```python
from build123d import *

# Parameters (mm, degrees)
SKETCH1_W_MOCK_PCB_W     = 63.5
SKETCH1_W_MOCK_PCB_H     = 209.042
BOSS_EXTRUDE1_DEPTH      = 6.35
F_5_16_CLEARANCE_HOLE1_D = 8.4328
CUT_EXTRUDE1_DEPTH       = 13.7


with BuildPart() as part:
    # Sketch1 w/mock PCB → Boss-Extrude1 (new body, symmetric)
    with BuildSketch(Plane.XY):
        Rectangle(SKETCH1_W_MOCK_PCB_W, SKETCH1_W_MOCK_PCB_H)
    extrude(amount=BOSS_EXTRUDE1_DEPTH, both=True)

    # 5/16 Clearance Hole1 (through all)
    with Locations(Plane.XY.offset(6.35)):
        with Locations((-19.05, -94.869), (19.05, -94.869)):
            Hole(F_5_16_CLEARANCE_HOLE1_D / 2)

    # Sketch3 → Cut-Extrude1 (cut, through all)
    with BuildSketch(Plane.XY.offset(6.35)):
        with BuildLine():
            Line((-23.2664, 93.599), (-23.2664, 96.139))
            ThreePointArc((-23.2664, 96.139), (-19.05, 100.3554), (-14.8336, 96.139))
            Line((-14.8336, 96.139), (-14.8336, 93.599))
            ThreePointArc((-14.8336, 93.599), (-19.05, 89.3826), (-23.2664, 93.599))
        make_face()
        with BuildLine():
            Line((23.2664, 93.599), (23.2664, 96.139))
            ThreePointArc((23.2664, 96.139), (19.05, 100.3554), (14.8336, 96.139))
            Line((14.8336, 96.139), (14.8336, 93.599))
            ThreePointArc((14.8336, 93.599), (19.05, 89.3826), (23.2664, 93.599))
        make_face()
    extrude(amount=-CUT_EXTRUDE1_DEPTH, mode=Mode.SUBTRACT)


solid = part.part
```
CAD build for the part. Positions are in the model's coordinates, mm. A direction names the side the tool comes from. Coordinates: 2 decimals unless noted, no trailing zeros. Order: outer loops, then holes, each group sorted by start corner. A loop starts at its lowest first (then second) coordinate and runs counter-clockwise, first axis right, second up.
(1) Saw through at B-B, the plane x = 20.5. Write the cut outline in (y, z).
Solution:
outline: (-104.52, -6.35) - (-98.83, -6.35) - (-98.83, 6.35) - (-104.52, 6.35) - close; (-90.91, -6.35) - (89.64, -6.35) - (89.64, 6.35) - (-90.91, 6.35) - close; (100.1, -6.35) - (104.52, -6.35) - (104.52, 6.35) - (100.1, 6.35) - close
(2) Which spindle directions (+Z, -Z, +X, -X, +Y, -Y) get a long thin tool onto all of the face, cutting with end or side? Do faces 1 (the face through (-18.957, 89.384, 0.089)), 2 (the face through (-31.75, -1, 0)). Say none if no direction does.
Solution:
face 1: +Z, -Z
face 2: +Z, -Z, -X, +Y, -Y
(3) Drill centre lines: L1, parallel to Y at x = -19.05, z = 3.25; L2, parallel to Y at x = -19.5, z = -5.5. Where is each one in solid material? Low to high.
Solution:
L1: y = -104.52 to -99.09, -90.65 to 89.38, 100.36 to 104.52
L2: y = -104.52 to -99.06, -90.68 to 89.41, 100.33 to 104.52
(4) Pin check, flat tip, straight feed: pin 1 Ø6.5 at (x, y) = (-19.05, -94.869) entering from -Z. Stop position of the tip, or through.
Solution:
pin 1: passes through
(5) Saw through at A-A, the plane x = -19.05. Write the cut outline in (y, z).
Solution:
outline: (-104.52, -6.35) - (-99.09, -6.35) - (-99.09, 6.35) - (-104.52, 6.35) - close; (-90.65, -6.35) - (89.38, -6.35) - (89.38, 6.35) - (-90.65, 6.35) - close; (100.36, -6.35) - (104.52, -6.35) - (104.52, 6.35) - (100.36, 6.35) - close
(6) Mould opens along Y. For faces 3 (the face through (19.143, 100.354, 0.089)), 4 (the face through (0, 1, 6.35)), 5 (the face through (18.957, 89.384, 0.089)), 6 (the face through (0, 104.521, 0)) say: released by +Y, released by -Y, zero draft, split by the parting line, or undercut.
Solution:
face 3: undercut
face 4: zero draft
face 5: undercut
face 6: released by +Y
